Verification items for this drawing (mm, ordinates from the low corner). A direction names the side the tool comes from. Coordinates: 2 decimals unless noted, no trailing zeros. Loops run counter-clockwise (first coordinate to the right, second up) from the corner with the lowest first, then second, coordinate; pieces in that order, holes last. Notation, with made-up numbers: M 3.25,36 L 33.25,36 A13 ccw 33.25,46 Z; hole C 71.25,32 d3. An arc over 180 degrees is marked long. Use CSV: the item, a comma, the result in double quotes.
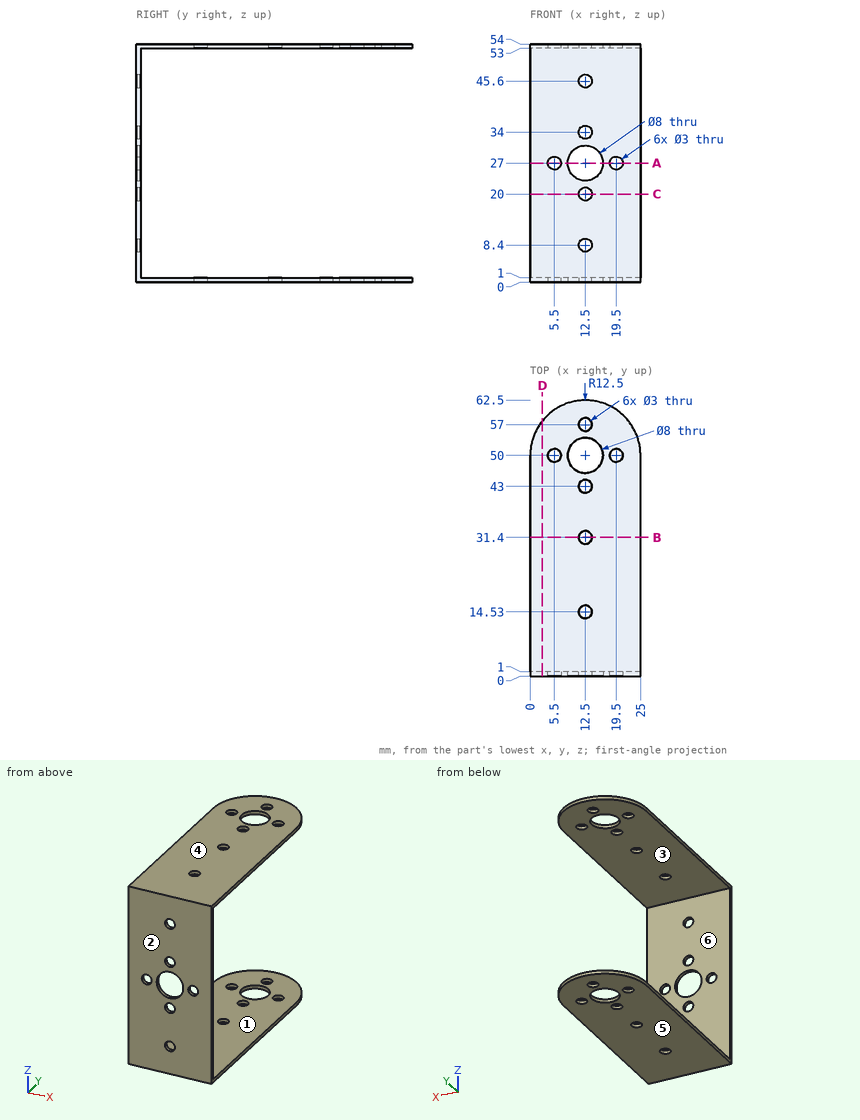
1. Gauge pin test, flat ends, axial feed: P1, Ø4, axis at x = 4, z = 40, coming from the +Y side; P2, Ø3.5, axis at x = 12.5, y = 57, coming from the +Z side. Record the tip position at first contact, or that the pin passes through.
The answers:
P1,"y = 1"
P2,"z = 54"
2. Thickness scan on line 1 (Y direction, x = 12.5, z = 53.7); line 2 (Z direction, x = 11.5, y = 21.5); line 3 (Y direction, x = 5.75, z = 49). Record the ranges inside material, lowest first. Write a range as [from, to].
The answers:
line 1,"[0, 13.03], [16.03, 29.9], [32.9, 41.5], [44.5, 46], [54, 55.5], [58.5, 62.5]"
line 2,"[0, 1], [53, 54]"
line 3,"[0, 1]"
3. Release check for a two-part mould opening along Z. For the marked faces 3, 4, 5 and 6 record: +Z half, -Z half, draft (parallel to the pull), parting line (faces both ways), or undercut.
The answers:
face 3,"undercut"
face 4,"+Z half"
face 5,"-Z half"
face 6,"undercut"
4. Section check A-A, the plane z = 27. Record the cut outline in (x, y).
The answers:
outline,"M 0,0 L 4,0 L 4,1 L 0,1 Z; M 7,0 L 8.5,0 L 8.5,1 L 7,1 Z; M 16.5,0 L 18,0 L 18,1 L 16.5,1 Z; M 21,0 L 25,0 L 25,1 L 21,1 Z"
5. Section check D-D, the plane x = 2.75. Record the cut outline in (y, z), plus the area to 3 significant figures.
The answers:
outline,"M 0,0 L 57.82,0 L 57.82,1 L 1,1 L 1,53 L 57.82,53 L 57.82,54 L 0,54 Z"
area,"168 mm^2"
6. Section check C-C, the plane z = 20. Record the cut outline in (x, y).
The answers:
outline,"M 0,0 L 11,0 L 11,1 L 0,1 Z; M 14,0 L 25,0 L 25,1 L 14,1 Z"
7. Section check B-B, the plane y = 31.4. Record the cut outline in (x, z), plus the area to 3 significant figures.
The answers:
outline,"M 0,0 L 11,0 L 11,1 L 0,1 Z; M 0,53 L 11,53 L 11,54 L 0,54 Z; M 14,0 L 25,0 L 25,1 L 14,1 Z; M 14,53 L 25,53 L 25,54 L 14,54 Z"
area,"44.0 mm^2"
8. Set-up check for the marked faces 1 and 2: record each of +Z, -Z, +X, -X, +Y, -Y from which the full face is reachable in a straight line by a thin tool's end or side.
The answers:
face 1,"+X, -X, +Y"
face 2,"+Z, -Z, +X, -X, -Y"
